Verification items for the finished model (mm, model axes). A direction names the side the tool comes from. Give positions to 0.01 mm unless a question says otherwise; leave off trailing zeros. Loops run counter-clockwise (first coordinate to the right, second up) from the corner with the lowest first, then second, coordinate; pieces in that order, holes last. Notation, with made-up numbers: (8.25, -16) - (14.25, -16) arc R22 cw to (14.25, 13) - close; hole circle Ø9 at (27, -17). An arc over 180 degrees is marked (long way). One line per question, with ' | ' between items. Start each with the question number.
1. Depth check by flat-ended pin: pin 1 Ø1.3 at (y, z) = (30, 1) entering from -X; pin 2 Ø2 at (x, z) = (-5.5, 3) entering from +Y; pin 3 Ø1.3 at (x, z) = (29, 2.5) entering from +Y. Enter the tip coordinate at first touch or a pass-through.
2. Section check A-A, the plane z = 1.7. State how many separate pieces and enclosed holes the cut face has, then the cut area to 3 significant figures.
3. Mould release check, pull along X, two halves, no side actions. Record for faces 1 (the face through (32.924, -0.861, 2.191)), 2 (the face through (9, -29, 2)), 3 (the face through (29, 9, 2)), 4 (the face through (-33.22, -1.37, 2.19)): +X half, -X half, draft (parallel to the pull), parting line (faces both ways), or undercut.
4. Section check B-B, the plane y = -35. Enter the section's corners in (x, z) (3 decimals).
5. Tool access check on faces 5 (the face through (-1.2, -33.1, 2.2)), 6 (the face through (-10, -3, 0)), 7 (the face through (-29, -9, 2)), 8 (the face through (9, 29, 2)), 9 (the face through (-29, 9, 2)). Record the directions out of +Z, -Z, +X, -X, +Y, -Y that give a thin tool (end or side, any length) a straight path to the whole face; none if there is none.
6. Section check D-D, the plane x = 12. Enter the section's corners in (y, z) (3 decimals), then the cut area to 3 significant figures.
7. Thickness scan on line 1 along Y through (x, z) = (0, 1.15); line 2 along X through (y, z) = (2, 2.4); line 3 along X through (y, z) = (24, 1.5). Record the ranges inside material, lowest first. Write a range as from..to.
from build123d import *

# Parameters (mm, degrees)
F0_W     = 84
F0_H     = 18
F1_DEPTH = 4.445
F2_W     = 18
F2_H     = 84
F3_DEPTH = 4.445
F4_R     = 8.89
F6_D     = 4.4958
F7_R     = 9.5
F8_DEPTH = 4.446
F9_R     = 15.24


with BuildPart() as f1:
    # F0 (on Top) → F1 (new body)
    with BuildSketch(Plane.XY):
        Rectangle(F0_W, F0_H)
    extrude(amount=F1_DEPTH)

    # F2 (on Top) → F3 (join, through all)
    with BuildSketch(Plane.XY):
        Rectangle(F2_W, F2_H)
    extrude(amount=F3_DEPTH)

    # F4
    f4_edges = [f1.edges().sort_by_distance(p)[0] for p in [
        (9, -42, 2.2225),
        (-9, -42, 2.2225),
        (42, -9, 2.2225),
        (42, 9, 2.2225),
        (9, 42, 2.2225),
        (-42, -9, 2.2225),
        (-42, 9, 2.2225),
        (-9, 42, 2.2225),
    ]]
    fillet(f4_edges, radius=F4_R)

    # F6 (through all)
    with Locations(Plane.XY.offset(4.445)):
        with Locations((35, 0), (0, -35), (-35, 0), (0, 35)):
            Hole(F6_D / 2)

    # F7 (on Top) → F8 (cut, through all)
    with BuildSketch(Plane.XY):
        Circle(F7_R)
    extrude(amount=F8_DEPTH, mode=Mode.SUBTRACT)

    # F9
    f9_edges = [f1.edges().sort_by_distance(p)[0] for p in [
        (9, 9, 2.2225),
        (9, -9, 2.2225),
        (-9, -9, 2.2225),
        (-9, 9, 2.2225),
    ]]
    fillet(f9_edges, radius=F9_R)


solid = f1.part
Results list:
1) pin 1: x = -9 | pin 2: y = 40.84 | pin 3: y = 9
2) separate pieces: 1 | enclosed holes: 5 | area: 2,420 mm²
3) face 1: undercut | face 2: +X half | face 3: draft | face 4: undercut
4) outline: (-8.797, 0) - (-2.248, 0) - (-2.248, 4.445) - (-8.797, 4.445) - close; (2.248, 0) - (8.797, 0) - (8.797, 4.445) - (2.248, 4.445) - close
5) face 5: +Z, -Z | face 6: -Z, +X, -X, +Y, -Y | face 7: +Z, -Z, -X, -Y | face 8: +Z, -Z, +X, +Y | face 9: +Z, -Z, -X, +Y
6) outline: (-15.16, 0) - (15.16, 0) - (15.16, 4.445) - (-15.16, 4.445) - close | area: 135 mm²
7) line 1: -42..-37.25, -32.75..-9.5, 9.5..32.75, 37.25..42 | line 2: -41.8..-36.03, -33.97..-9.29, 9.29..33.97, 36.03..41.8 | line 3: -9..9
